from build123d import *

# Parameters (mm, degrees)
SKETCH_1_W          = 56
SKETCH_1_H          = 20
EXTRUDE_1_DEPTH     = 2
CUT_EXTRUDE_1_REACH = 4
SKETCH_2_R          = 3
SKETCH_2_R_2        = 1.5
EXTRUDE_2_DEPTH     = 2
SKETCH_4_R          = 4
SKETCH_4_R_2        = 1.5
CUT_EXTRUDE_2_DEPTH = 2


with BuildPart() as part:
    # 草图1 → 凸台-拉伸1 (new body)
    with BuildSketch(Plane(origin=(0, 0, 0), x_dir=(1, 0, 0), z_dir=(0, 1, 0))):
        with Locations((28, 10)):
            Rectangle(SKETCH_1_W, SKETCH_1_H)
    extrude(amount=EXTRUDE_1_DEPTH)

    # 草图2 → 切除-拉伸1 (cut, up to next)
    with BuildSketch(Plane(origin=(0, 2, 0), x_dir=(1, 0, 0), z_dir=(0, 1, 0)), mode=Mode.PRIVATE) as cut_extrude_1_sk1:
        with Locations((28, 10)):
            Circle(SKETCH_2_R)
    cut_extrude_1_tool1 = extrude(cut_extrude_1_sk1.sketch, amount=-CUT_EXTRUDE_1_REACH, mode=Mode.PRIVATE) & part.part
    add(cut_extrude_1_tool1.solids().sort_by_distance((28, 2, -10))[0], mode=Mode.SUBTRACT)
    # 草图2 → 切除-拉伸1 (cut, up to next)
    with BuildSketch(Plane(origin=(0, 2, 0), x_dir=(1, 0, 0), z_dir=(0, 1, 0)), mode=Mode.PRIVATE) as cut_extrude_1_sk2:
        with Locations((32.949747468, 5.050252532)):
            Circle(SKETCH_2_R_2)
    cut_extrude_1_tool2 = extrude(cut_extrude_1_sk2.sketch, amount=-CUT_EXTRUDE_1_REACH, mode=Mode.PRIVATE) & part.part
    add(cut_extrude_1_tool2.solids().sort_by_distance((32.949747, 2, -5.050253))[0], mode=Mode.SUBTRACT)
    # 草图2 → 切除-拉伸1 (cut, up to next)
    with BuildSketch(Plane(origin=(0, 2, 0), x_dir=(1, 0, 0), z_dir=(0, 1, 0)), mode=Mode.PRIVATE) as cut_extrude_1_sk3:
        with Locations((23.050252532, 5.050252532)):
            Circle(SKETCH_2_R_2)
    cut_extrude_1_tool3 = extrude(cut_extrude_1_sk3.sketch, amount=-CUT_EXTRUDE_1_REACH, mode=Mode.PRIVATE) & part.part
    add(cut_extrude_1_tool3.solids().sort_by_distance((23.050253, 2, -5.050253))[0], mode=Mode.SUBTRACT)
    # 草图2 → 切除-拉伸1 (cut, up to next)
    with BuildSketch(Plane(origin=(0, 2, 0), x_dir=(1, 0, 0), z_dir=(0, 1, 0)), mode=Mode.PRIVATE) as cut_extrude_1_sk4:
        with Locations((23.050252532, 14.949747468)):
            Circle(SKETCH_2_R_2)
    cut_extrude_1_tool4 = extrude(cut_extrude_1_sk4.sketch, amount=-CUT_EXTRUDE_1_REACH, mode=Mode.PRIVATE) & part.part
    add(cut_extrude_1_tool4.solids().sort_by_distance((23.050253, 2, -14.949747))[0], mode=Mode.SUBTRACT)
    # 草图2 → 切除-拉伸1 (cut, up to next)
    with BuildSketch(Plane(origin=(0, 2, 0), x_dir=(1, 0, 0), z_dir=(0, 1, 0)), mode=Mode.PRIVATE) as cut_extrude_1_sk5:
        with Locations((32.949747468, 14.949747468)):
            Circle(SKETCH_2_R_2)
    cut_extrude_1_tool5 = extrude(cut_extrude_1_sk5.sketch, amount=-CUT_EXTRUDE_1_REACH, mode=Mode.PRIVATE) & part.part
    add(cut_extrude_1_tool5.solids().sort_by_distance((32.949747, 2, -14.949747))[0], mode=Mode.SUBTRACT)
    # 草图2 → 切除-拉伸1 (cut, up to next)
    with BuildSketch(Plane(origin=(0, 2, 0), x_dir=(1, 0, 0), z_dir=(0, 1, 0)), mode=Mode.PRIVATE) as cut_extrude_1_sk6:
        with Locations((13.150757595, 14.949747468)):
            Circle(SKETCH_2_R_2)
    cut_extrude_1_tool6 = extrude(cut_extrude_1_sk6.sketch, amount=-CUT_EXTRUDE_1_REACH, mode=Mode.PRIVATE) & part.part
    add(cut_extrude_1_tool6.solids().sort_by_distance((13.150758, 2, -14.949747))[0], mode=Mode.SUBTRACT)
    # 草图2 → 切除-拉伸1 (cut, up to next)
    with BuildSketch(Plane(origin=(0, 2, 0), x_dir=(1, 0, 0), z_dir=(0, 1, 0)), mode=Mode.PRIVATE) as cut_extrude_1_sk7:
        with Locations((13.150757595, 5.050252532)):
            Circle(SKETCH_2_R_2)
    cut_extrude_1_tool7 = extrude(cut_extrude_1_sk7.sketch, amount=-CUT_EXTRUDE_1_REACH, mode=Mode.PRIVATE) & part.part
    add(cut_extrude_1_tool7.solids().sort_by_distance((13.150758, 2, -5.050253))[0], mode=Mode.SUBTRACT)
    # 草图2 → 切除-拉伸1 (cut, up to next)
    with BuildSketch(Plane(origin=(0, 2, 0), x_dir=(1, 0, 0), z_dir=(0, 1, 0)), mode=Mode.PRIVATE) as cut_extrude_1_sk8:
        with Locations((42.849242405, 5.050252532)):
            Circle(SKETCH_2_R_2)
    cut_extrude_1_tool8 = extrude(cut_extrude_1_sk8.sketch, amount=-CUT_EXTRUDE_1_REACH, mode=Mode.PRIVATE) & part.part
    add(cut_extrude_1_tool8.solids().sort_by_distance((42.849242, 2, -5.050253))[0], mode=Mode.SUBTRACT)
    # 草图2 → 切除-拉伸1 (cut, up to next)
    with BuildSketch(Plane(origin=(0, 2, 0), x_dir=(1, 0, 0), z_dir=(0, 1, 0)), mode=Mode.PRIVATE) as cut_extrude_1_sk9:
        with Locations((42.849242405, 14.949747468)):
            Circle(SKETCH_2_R_2)
    cut_extrude_1_tool9 = extrude(cut_extrude_1_sk9.sketch, amount=-CUT_EXTRUDE_1_REACH, mode=Mode.PRIVATE) & part.part
    add(cut_extrude_1_tool9.solids().sort_by_distance((42.849242, 2, -14.949747))[0], mode=Mode.SUBTRACT)

    # 草图3 → 凸台-拉伸2 (add)
    with BuildSketch(Plane.ZY):
        with BuildLine():
            Line((-20, 2), (0, 2))
            Line((0, 2), (0, 27))
            ThreePointArc((0, 27), (-10, 37), (-20, 27))
            Line((-20, 27), (-20, 2))
        make_face()
    extrude_2 = extrude(amount=-EXTRUDE_2_DEPTH)

    # 草图4 → 切除-拉伸2 (cut)
    with BuildSketch(Plane.ZY):
        with Locations((-10, 27)):
            Circle(SKETCH_4_R)
        with Locations((-10, 34)):
            Circle(SKETCH_4_R_2)
        with Locations((-3, 27)):
            Circle(SKETCH_4_R_2)
        with Locations((-5.050252532, 22.050252532)):
            Circle(SKETCH_4_R_2)
        with Locations((-10, 20)):
            Circle(SKETCH_4_R_2)
        with Locations((-14.949747468, 22.050252532)):
            Circle(SKETCH_4_R_2)
        with Locations((-17, 27)):
            Circle(SKETCH_4_R_2)
    cut_extrude_2 = extrude(amount=-CUT_EXTRUDE_2_DEPTH, mode=Mode.SUBTRACT)

    # 镜向1: 凸台-拉伸2, 切除-拉伸2 across plane
    add(extrude_2.mirror(Plane.ZY.offset(-28)))
    add(cut_extrude_2.mirror(Plane.ZY.offset(-28)), mode=Mode.SUBTRACT)


solid = part.part
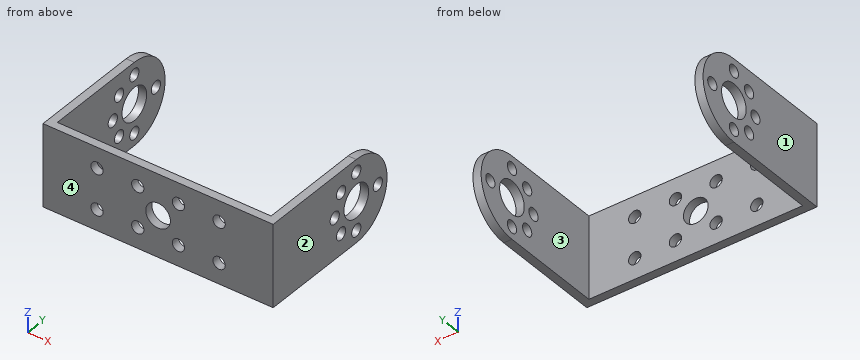
Geometry: final body of the model. Coordinates: model frame, mm. Face numbers are marked on the shaded views. Give positions to 0.01 mm unless a question says otherwise; leave off trailing zeros. Write each loop counter-clockwise with the first axis right and the second up, starting at its lowest first coordinate (ties: lowest second). Pieces come first, ordered by that corner, then holes. Notation, with made-up numbers: (47.5, -36) - (54.5, -36) arc R14 ccw to (54.5, -25) - close; hole circle Ø11 at (-18, 21.5). An arc over 180 degrees is marked (long way). Return JSON: item names as keys, results as strings. Group by question number.
1) Mould query, pull axis X, two halves, no side actions, for the marked faces 1, 2, 3 and 4. Classes: released by +X, released by -X, zero draft, split by the parting line, or undercut.
2) Section D-D on x = 8.5. Return the cut outline in (y, z), plus the area to 3 significant figures.
3) Section A-A on x = 28. Return the cut outline in (y, z), plus the area to 3 significant figures.
4) Section B-B on y = 30. Return the cut outline in (x, z).
5) First-contact query: P1, Ø10, axis at x = 26.5, z = -12, coming from the +Y side; P2, Ø1.8, axis at y = 27, z = -3, coming from the +X side. Flat tips, straight axial feed; report the tip coordinate or a pass-through.
6) Line query: line 1 (Y direction, x = 55.5, z = -10); line 2 (X direction, y = 7, z = -16.75); line 3 (X direction, y = 0.75, z = -10). Output: solid intervals per line, ascending.
7) Section C-C on z = -10. State how many separate pieces and enclosed holes the cut face has, plus the area to 3 significant figures.
Filled in:
{
 "1": {"face 1": "released by -X", "face 2": "released by +X", "face 3": "undercut", "face 4": "zero draft"},
 "2": {"outline": "(0, -20) - (2, -20) - (2, 0) - (0, 0) - close", "area": "40.0 mm^2"},
 "3": {"outline": "(0, -20) - (2, -20) - (2, -13) - (0, -13) - close; (0, -7) - (2, -7) - (2, 0) - (0, 0) - close", "area": "28.0 mm^2"},
 "4": {"outline": "(0, -19.54) - (2, -19.54) - (2, -12.65) - (0, -12.65) - close; (0, -7.35) - (2, -7.35) - (2, -0.46) - (0, -0.46) - close; (54, -19.54) - (56, -19.54) - (56, -12.65) - (54, -12.65) - close; (54, -7.35) - (56, -7.35) - (56, -0.46) - (54, -0.46) - close"},
 "5": {"P1": "stops at y = 2", "P2": "passes through"},
 "6": {"line 1": "y = 0 to 18.5, 21.5 to 23, 31 to 32.5, 35.5 to 37", "line 2": "x = 0 to 2, 54 to 56", "line 3": "x = 0 to 25, 31 to 56"},
 "7": {"separate pieces": "8", "enclosed holes": "0", "area": "184 mm^2"}
}
